Read the model definition and answer for the solid it produces. Units are mm, in the model's axes. Coordinates: 2 decimals unless noted, no trailing zeros. Write each loop counter-clockwise with the first axis right and the second up, starting at its lowest first coordinate (ties: lowest second). Pieces come first, ordered by that corner, then holes.
(1) The part is cut by section B-B, the plane x = 4. Determine the outline of the cut face in (y, z), and give its area (3 significant figures).
(2) The part is cut by section C-C, the plane z = 17.5. Determine the outline of the cut face in (x, y), and give its area (3 significant figures).
(3) The part is cut by section A-A, the plane z = -70. Determine the outline of the cut face in (x, y).
(4) The part is cut by section D-D, the plane y = 2. State how many separate pieces and enclosed holes the cut face has, and give its area (3 significant figures).
(5) Straight lines are drawn through the part: line 1 along X through (y, z) = (0.2, 10); line 2 along Z through (x, y) = (137.5, 2.5); line 3 along Z through (x, y) = (-77.5, 1.8). For each, find the intervals that lie inside material, in ascending order.
```python
from build123d import *

# Parameters (mm, degrees)
SKETCH1_W                 = 320
SKETCH1_H                 = 213
OUTER_PROFILE_DEPTH       = 3
SKETCH5_W                 = 52
SKETCH5_H                 = 35
CUTOUT_DEPTH              = 193.227079258
CORNER_RAD_R              = 5
LPATTERN1_COUNT           = 5
LPATTERN1_PITCH           = 59
LPATTERN1_COUNT_DIR2      = 4
LPATTERN1_PITCH_DIR2      = 42
CORNER_RAD_OF_LPATTERN1_R = 5
CORNER_DEPTH              = 193.227079258
CORNERSB_COPY_1_DEPTH     = 193.227079258
SKETCH7_W                 = 135
SKETCH7_H                 = 35
CUT_EXTRUDE2_DEPTH        = 193.227079398


with BuildPart() as part:
    # Sketch1 → Outer Profile (new body)
    with BuildSketch(Plane(origin=(0, 0, 0), x_dir=(1, 0, 0), z_dir=(0, 1, 0))):
        Rectangle(SKETCH1_W, SKETCH1_H)
    extrude(amount=OUTER_PROFILE_DEPTH)

    # Sketch5 → Cutout (cut, through all)
    with BuildSketch(Plane(origin=(0, 3, 0), x_dir=(1, 0, 0), z_dir=(0, 1, 0))):
        with Locations((-118, -58.5)):
            Rectangle(SKETCH5_W, SKETCH5_H)
    cutout = extrude(amount=-CUTOUT_DEPTH, mode=Mode.SUBTRACT)

    # Corner Rad
    corner_rad_edges = [part.edges().sort_by_distance(p)[0] for p in [
        (-144, 1.5, 76),
        (-144, 1.5, 41),
        (-92, 1.5, 41),
        (-92, 1.5, 76),
    ]]
    fillet(corner_rad_edges, radius=CORNER_RAD_R)

    # LPattern1: Cutout 5 × 4
    with Locations(*[(i * LPATTERN1_PITCH, 0, -j * LPATTERN1_PITCH_DIR2) for i in range(LPATTERN1_COUNT) for j in range(LPATTERN1_COUNT_DIR2) if (i, j) != (0, 0)]):
        add(cutout, mode=Mode.SUBTRACT)

    # Corner Rad of LPattern1
    corner_rad_of_lpattern1_edges = [part.edges().sort_by_distance(p)[0] for p in [
        (-144, 1.5, 34),
        (-144, 1.5, -1),
        (-92, 1.5, -1),
        (-92, 1.5, 34),
        (-144, 1.5, -8),
        (-144, 1.5, -43),
        (-92, 1.5, -43),
        (-92, 1.5, -8),
        (-144, 1.5, -50),
        (-144, 1.5, -85),
        (-92, 1.5, -85),
        (-92, 1.5, -50),
        (-85, 1.5, 76),
        (-85, 1.5, 41),
        (-33, 1.5, 41),
        (-33, 1.5, 76),
        (-85, 1.5, 34),
        (-85, 1.5, -1),
        (-33, 1.5, -1),
        (-33, 1.5, 34),
        (-85, 1.5, -8),
        (-85, 1.5, -43),
        (-33, 1.5, -43),
        (-33, 1.5, -8),
        (-85, 1.5, -50),
        (-85, 1.5, -85),
        (-33, 1.5, -85),
        (-33, 1.5, -50),
        (-26, 1.5, 76),
        (-26, 1.5, 41),
        (26, 1.5, 41),
        (26, 1.5, 76),
        (-26, 1.5, 34),
        (-26, 1.5, -1),
        (26, 1.5, -1),
        (26, 1.5, 34),
        (-26, 1.5, -8),
        (-26, 1.5, -43),
        (26, 1.5, -43),
        (26, 1.5, -8),
        (-26, 1.5, -50),
        (-26, 1.5, -85),
        (26, 1.5, -85),
        (26, 1.5, -50),
        (33, 1.5, 76),
        (33, 1.5, 41),
        (85, 1.5, 41),
        (85, 1.5, 76),
        (33, 1.5, 34),
        (33, 1.5, -1),
        (85, 1.5, -1),
        (85, 1.5, 34),
        (33, 1.5, -8),
        (33, 1.5, -43),
        (85, 1.5, -43),
        (85, 1.5, -8),
        (33, 1.5, -50),
        (33, 1.5, -85),
        (85, 1.5, -85),
        (85, 1.5, -50),
        (92, 1.5, 76),
        (92, 1.5, 41),
        (144, 1.5, 41),
        (144, 1.5, 76),
        (92, 1.5, 34),
        (92, 1.5, -1),
        (144, 1.5, -1),
        (144, 1.5, 34),
        (92, 1.5, -8),
        (92, 1.5, -43),
        (144, 1.5, -43),
        (144, 1.5, -8),
        (92, 1.5, -50),
        (92, 1.5, -85),
        (144, 1.5, -85),
        (144, 1.5, -50),
    ]]
    fillet(corner_rad_of_lpattern1_edges, radius=CORNER_RAD_OF_LPATTERN1_R)

    # Sketch6 → Corner (cut, through all)
    with BuildSketch(Plane(origin=(0, 3, 0), x_dir=(1, 0, 0), z_dir=(0, 1, 0))):
        with BuildLine():
            Line((-135, 106.5), (-160, 106.5))
            Line((-160, 106.5), (-160, 91.5))
            add(Edge.make_bspline(
                [(-135, 106.5), (-160, 106.5), (-160, 91.5)],
                knots=[1.570796327, 1.570796327, 1.570796327, 3.141592654, 3.141592654, 3.141592654], degree=2, weights=[1, 0.707106781, 1]))
        make_face()
    corner = extrude(amount=-CORNER_DEPTH, mode=Mode.SUBTRACT)

    # CornersA: Corner across plane
    add(corner.mirror(Plane(origin=(0, 0, 0), x_dir=(0, 0, 1), z_dir=(1, 0, 0))), mode=Mode.SUBTRACT)

    # CornersB: Corner across plane
    add(corner.mirror(Plane.XY), mode=Mode.SUBTRACT)

    # CornersB copy 1 sketch → CornersB copy 1 (cut, through all)
    with BuildSketch(Plane(origin=(0, 3, 0), x_dir=(-1, 0, 0), z_dir=(0, 1, 0))):
        with BuildLine():
            Line((-135, 106.5), (-160, 106.5))
            Line((-160, 106.5), (-160, 91.5))
            add(Edge.make_bspline(
                [(-135, 106.5), (-160, 106.5), (-160, 91.5)],
                knots=[1.570796327, 1.570796327, 1.570796327, 3.141592654, 3.141592654, 3.141592654], degree=2, weights=[1, 0.707106781, 1]))
        make_face()
    extrude(amount=-CORNERSB_COPY_1_DEPTH, mode=Mode.SUBTRACT)

    # Sketch7 → Cut-Extrude2 (cut, through all)
    with BuildSketch(Plane(origin=(0, 3, 0), x_dir=(1, 0, 0), z_dir=(0, 1, 0))):
        with Locations((-29.5, 67.5)):
            Rectangle(SKETCH7_W, SKETCH7_H)
    extrude(amount=-CUT_EXTRUDE2_DEPTH, mode=Mode.SUBTRACT)


solid = part.part
```
Computed:
1. outline: (0, -106.5) - (3, -106.5) - (3, -85) - (0, -85) - close; (0, -50) - (3, -50) - (3, -43) - (0, -43) - close; (0, -8) - (3, -8) - (3, -1) - (0, -1) - close; (0, 34) - (3, 34) - (3, 41) - (0, 41) - close; (0, 76) - (3, 76) - (3, 106.5) - (0, 106.5) - close
1. area: 219 mm2
2. outline: (-160, 0) - (-144, 0) - (-144, 3) - (-160, 3) - close; (-92, 0) - (-85, 0) - (-85, 3) - (-92, 3) - close; (-33, 0) - (-26, 0) - (-26, 3) - (-33, 3) - close; (26, 0) - (33, 0) - (33, 3) - (26, 3) - close; (85, 0) - (92, 0) - (92, 3) - (85, 3) - close; (144, 0) - (160, 0) - (160, 3) - (144, 3) - close
2. area: 180 mm2
3. outline: (-160, 0) - (-144, 0) - (-144, 3) - (-160, 3) - close; (85, 0) - (92, 0) - (92, 3) - (85, 3) - close; (144, 0) - (160, 0) - (160, 3) - (144, 3) - close
4. separate pieces: 1
4. enclosed holes: 17
4. area: 31,100 mm2
5. line 1: x = -160 to -144, -92 to -85, -33 to -26, 26 to 33, 85 to 92, 144 to 160
5. line 2: z = -106.42 to -85, -50 to -43, -8 to -1, 34 to 41, 76 to 106.42
5. line 3: z = -106.5 to -85, -50 to -43, -8 to -1, 34 to 41, 76 to 106.5
